Geometry: see drawing. Coordinates: mm, zero at the bounding-box minimum. A direction names the side the tool comes from. Give positions to 0.01 mm unless a question says otherwise; leave off trailing zeros. Loops run counter-clockwise (first coordinate to the right, second up) from the corner with the lowest first, then second, coordinate; pieces in that order, holes last. Notation, with made-up numbers: M 51.5,44.5 L 65.5,44.5 A21 cw 65.5,63.5 Z; hole C 24,5 d10. An arc over 180 degrees is marked long. Put each result on its own line as item: value.
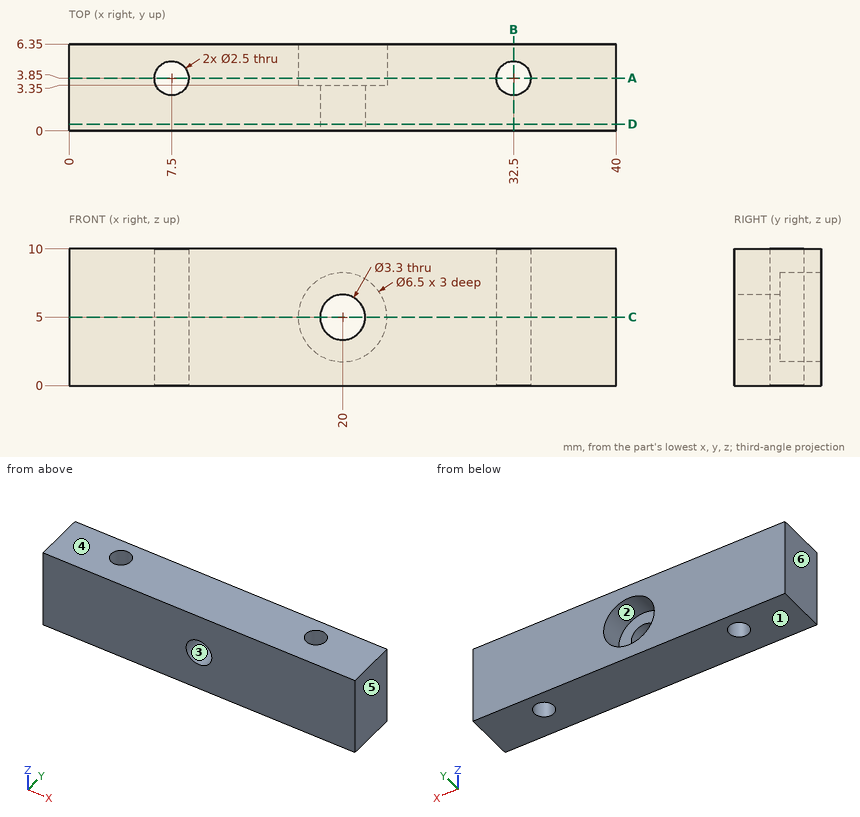
Item 1: Pin query (flat end, axial travel): pin 1 Ø5 at (x, z) = (20, 5) entering from -Y. Return the tip coordinate at first contact, or that it passes through.
Output values:
pin 1: y = 0
Item 2: Section A-A on y = 3.85. Output: boundary loops of the cut face in (x, z).
Output values:
outline: M 0,0 L 6.25,0 L 6.25,10 L 0,10 Z; M 8.75,0 L 31.25,0 L 31.25,10 L 8.75,10 Z; M 33.75,0 L 40,0 L 40,10 L 33.75,10 Z; hole C 20,5 d6.5
Item 3: Section B-B on x = 32.5. Output: boundary loops of the cut face in (y, z), then the cut area to 3 significant figures.
Output values:
outline: M 0,0 L 2.6,0 L 2.6,10 L 0,10 Z; M 5.1,0 L 6.35,0 L 6.35,10 L 5.1,10 Z
area: 38.5 mm²
Item 4: Set-up query: the marked faces 1 and 2. Return all of +Z, -Z, +X, -X, +Y, -Y with unobstructed straight access to the full face (end or side cutting, diameter ignored); none if empty.
Output values:
face 1: -Z, +X, -X, +Y, -Y
face 2: +Y
Item 5: Line query: probe 1 along Y at (x, z) = (32.5, 5); probe 2 along X at (y, z) = (1.45, 5); probe 3 along Z at (x, y) = (20, 4.55). Output: solid intervals per line, ascending. Write a range as [from, to].
Output values:
probe 1: [0, 2.6], [5.1, 6.35]
probe 2: [0, 18.35], [21.65, 40]
probe 3: [0, 1.75], [8.25, 10]
Item 6: Section D-D on y = 0.5. Output: boundary loops of the cut face in (x, z), then the cut area to 3 significant figures.
Output values:
outline: M 0,0 L 40,0 L 40,10 L 0,10 Z; hole C 20,5 d3.3
area: 391 mm²
Item 7: Section C-C on z = 5. Output: boundary loops of the cut face in (x, y), then the cut area to 3 significant figures.
Output values:
outline: M 0,0 L 18.35,0 L 18.35,3.35 L 16.75,3.35 L 16.75,6.35 L 0,6.35 Z; M 21.65,0 L 40,0 L 40,6.35 L 23.25,6.35 L 23.25,3.35 L 21.65,3.35 Z; hole C 7.5,3.85 d2.5; hole C 32.5,3.85 d2.5
area: 214 mm²
Item 8: Mould query, pull axis X, two halves, no side actions, for the marked faces 3, 4, 5 and 6. Classes: pulls with the +X half, pulls with the -X half, needs draft (parallel to the pull), parting line crosses it, or undercut.
Output values:
face 3: undercut
face 4: needs draft
face 5: pulls with the +X half
face 6: pulls with the -X half
